```python
from build123d import *

# Parameters (mm, degrees)
BOSS_EXTRUDE1_DEPTH = 16
CUT_EXTRUDE1_DEPTH  = 16
FILLET1_R           = 0.4
FILLET2_R           = 0.4
FILLET3_R           = 0.4
FILLET4_R           = 0.4
FILLET5_R           = 6.2
FILLET6_R           = 6.2
FILLET7_R           = 6.2
FILLET8_R           = 6.2
FILLET9_R           = 0.1
FILLET10_R          = 0.1
FILLET11_R          = 0.1
FILLET12_R          = 0.1
FILLET13_R          = 0.1
FILLET14_R          = 0.1
FILLET15_R          = 0.1
FILLET16_R          = 0.1
FILLET17_R          = 0.1
FILLET18_R          = 0.1
FILLET19_R          = 0.1
FILLET20_R          = 0.1
FILLET21_R          = 0.1
FILLET22_R          = 0.1
FILLET23_R          = 0.1
FILLET24_R          = 0.1


with BuildPart() as part:
    # Sketch1 → Boss-Extrude1 (new body)
    with BuildSketch(Plane.XY):
        with BuildLine():
            Line((-1.085, -1.085), (-1.085, -2.903924069))
            ThreePointArc((-1.085, -2.903924069), (0, -3.1), (1.085, -2.903924069))
            Line((1.085, -2.903924069), (1.085, -1.085))
            Line((1.085, -1.085), (2.903924069, -1.085))
            ThreePointArc((2.903924069, -1.085), (3.1, 0), (2.903924069, 1.085))
            Line((2.903924069, 1.085), (1.085, 1.085))
            Line((1.085, 1.085), (1.085, 2.903924069))
            ThreePointArc((1.085, 2.903924069), (0, 3.1), (-1.085, 2.903924069))
            Line((-1.085, 2.903924069), (-1.085, 1.085))
            Line((-1.085, 1.085), (-2.903924069, 1.085))
            ThreePointArc((-2.903924069, 1.085), (-3.1, 0), (-2.903924069, -1.085))
            Line((-2.903924069, -1.085), (-1.085, -1.085))
        make_face()
    extrude(amount=BOSS_EXTRUDE1_DEPTH)

    # Sketch2 → Cut-Extrude1 (cut)
    with BuildSketch(Plane.XY):
        with BuildLine():
            Line((0.84, -0.84), (2.248199279, -0.84))
            ThreePointArc((2.248199279, -0.84), (2.4, 0), (2.248199279, 0.84))
            Line((2.248199279, 0.84), (0.84, 0.84))
            Line((0.84, 0.84), (0.84, 2.248199279))
            ThreePointArc((0.84, 2.248199279), (0, 2.4), (-0.84, 2.248199279))
            Line((-0.84, 2.248199279), (-0.84, 0.84))
            Line((-0.84, 0.84), (-2.248199279, 0.84))
            ThreePointArc((-2.248199279, 0.84), (-2.4, 0), (-2.248199279, -0.84))
            Line((-2.248199279, -0.84), (-0.84, -0.84))
            Line((-0.84, -0.84), (-0.84, -2.248199279))
            ThreePointArc((-0.84, -2.248199279), (0, -2.4), (0.84, -2.248199279))
            Line((0.84, -2.248199279), (0.84, -0.84))
        make_face()
    extrude(amount=CUT_EXTRUDE1_DEPTH, mode=Mode.SUBTRACT)

    # Fillet1
    fillet1_edges = [part.edges().sort_by_distance(p)[0] for p in [
        (-0.84, 0.84, 8),
    ]]
    fillet(fillet1_edges, radius=FILLET1_R)

    # Fillet2
    fillet2_edges = [part.edges().sort_by_distance(p)[0] for p in [
        (0.84, 0.84, 8),
    ]]
    fillet(fillet2_edges, radius=FILLET2_R)

    # Fillet3
    fillet3_edges = [part.edges().sort_by_distance(p)[0] for p in [
        (0.84, -0.84, 8),
    ]]
    fillet(fillet3_edges, radius=FILLET3_R)

    # Fillet4
    fillet4_edges = [part.edges().sort_by_distance(p)[0] for p in [
        (-0.84, -0.84, 8),
    ]]
    fillet(fillet4_edges, radius=FILLET4_R)

    # Fillet5
    # the kernel refuses this fillet: 6.2 mm, written as the material it adds along each edge
    with BuildSketch(Plane(origin=(-1.085, 1.085, 0), x_dir=(-1, 0, 0), z_dir=(0, 0, 1))) as fillet5_piece_1:
        with BuildLine():
            CenterArc((5.198154004, -5.198154004), FILLET5_R, 123.027198012, 23.945603977)
            Line((0, -1.818924069), (0, 0))
            Line((0, 0), (1.818924069, 0))
        make_face()
    extrude(amount=16)

    # Fillet6
    # the kernel refuses this fillet: 6.2 mm, written as the material it adds along each edge
    with BuildSketch(Plane(origin=(-1.085, -1.085, 0), x_dir=(-1, 0, 0), z_dir=(0, 0, 1))) as fillet6_piece_1:
        with BuildLine():
            CenterArc((5.198154004, 5.198154004), FILLET6_R, 213.027198012, 23.945603977)
            Line((0, 1.818924069), (0, 0))
            Line((0, 0), (1.818924069, 0))
        make_face()
    extrude(amount=16)

    # Fillet7
    # the kernel refuses this fillet: 6.2 mm, written as the material it adds along each edge
    with BuildSketch(Plane(origin=(1.085, -1.085, 0), x_dir=(0, -1, 0), z_dir=(0, 0, 1))) as fillet7_piece_1:
        with BuildLine():
            CenterArc((5.198154004, 5.198154004), FILLET7_R, 213.027198012, 23.945603977)
            Line((0, 1.818924069), (0, 0))
            Line((0, 0), (1.818924069, 0))
        make_face()
    extrude(amount=16)

    # Fillet8
    # the kernel refuses this fillet: 6.2 mm, written as the material it adds along each edge
    with BuildSketch(Plane(origin=(1.085, 1.085, 0), x_dir=(1, 0, 0), z_dir=(0, 0, 1))) as fillet8_piece_1:
        with BuildLine():
            CenterArc((5.198154004, 5.198154004), FILLET8_R, 213.027198012, 23.945603977)
            Line((0, 1.818924069), (0, 0))
            Line((0, 0), (1.818924069, 0))
        make_face()
    extrude(amount=16)

    # Fillet9
    fillet9_edges = [part.edges().sort_by_distance(p)[0] for p in [
        (0.84, 2.248199279, 8),
    ]]
    fillet(fillet9_edges, radius=FILLET9_R)

    # Fillet10
    fillet10_edges = [part.edges().sort_by_distance(p)[0] for p in [
        (1.085, 2.903924069, 8),
    ]]
    fillet(fillet10_edges, radius=FILLET10_R)

    # Fillet11
    fillet11_edges = [part.edges().sort_by_distance(p)[0] for p in [
        (-1.085, 2.903924069, 8),
    ]]
    fillet(fillet11_edges, radius=FILLET11_R)

    # Fillet12
    fillet12_edges = [part.edges().sort_by_distance(p)[0] for p in [
        (-2.903924069, 1.085, 8),
    ]]
    fillet(fillet12_edges, radius=FILLET12_R)

    # Fillet13
    fillet13_edges = [part.edges().sort_by_distance(p)[0] for p in [
        (-2.903924069, -1.085, 8),
    ]]
    fillet(fillet13_edges, radius=FILLET13_R)

    # Fillet14
    fillet14_edges = [part.edges().sort_by_distance(p)[0] for p in [
        (-1.085, -2.903924069, 8),
    ]]
    fillet(fillet14_edges, radius=FILLET14_R)

    # Fillet15
    fillet15_edges = [part.edges().sort_by_distance(p)[0] for p in [
        (1.085, -2.903924069, 8),
    ]]
    fillet(fillet15_edges, radius=FILLET15_R)

    # Fillet16
    fillet16_edges = [part.edges().sort_by_distance(p)[0] for p in [
        (2.903924069, -1.085, 8),
    ]]
    fillet(fillet16_edges, radius=FILLET16_R)

    # Fillet17
    fillet17_edges = [part.edges().sort_by_distance(p)[0] for p in [
        (2.903924069, 1.085, 8),
    ]]
    fillet(fillet17_edges, radius=FILLET17_R)

    # Fillet18
    fillet18_edges = [part.edges().sort_by_distance(p)[0] for p in [
        (0.84, -2.248199279, 8),
    ]]
    fillet(fillet18_edges, radius=FILLET18_R)

    # Fillet19
    fillet19_edges = [part.edges().sort_by_distance(p)[0] for p in [
        (-0.84, -2.248199279, 8),
    ]]
    fillet(fillet19_edges, radius=FILLET19_R)

    # Fillet20
    fillet20_edges = [part.edges().sort_by_distance(p)[0] for p in [
        (-2.248199279, 0.84, 8),
    ]]
    fillet(fillet20_edges, radius=FILLET20_R)

    # Fillet21
    fillet21_edges = [part.edges().sort_by_distance(p)[0] for p in [
        (-2.248199279, -0.84, 8),
    ]]
    fillet(fillet21_edges, radius=FILLET21_R)

    # Fillet22
    fillet22_edges = [part.edges().sort_by_distance(p)[0] for p in [
        (-0.84, 2.248199279, 8),
    ]]
    fillet(fillet22_edges, radius=FILLET22_R)

    # Fillet23
    fillet23_edges = [part.edges().sort_by_distance(p)[0] for p in [
        (2.248199279, -0.84, 8),
    ]]
    fillet(fillet23_edges, radius=FILLET23_R)

    # Fillet24
    fillet24_edges = [part.edges().sort_by_distance(p)[0] for p in [
        (2.248199279, 0.84, 8),
    ]]
    fillet(fillet24_edges, radius=FILLET24_R)


solid = part.part
```
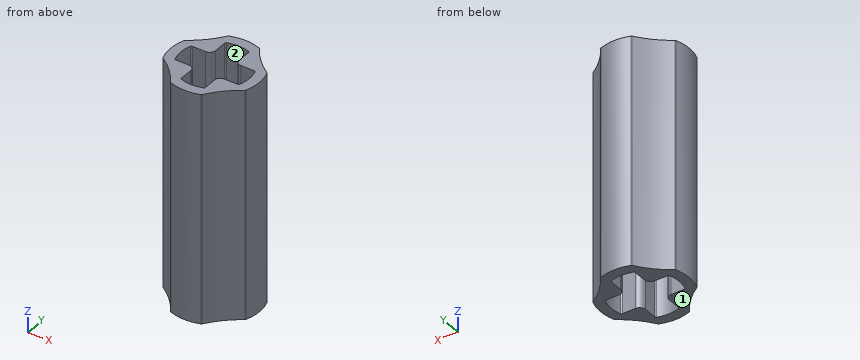
Here's how the part is built. I have some questions about the finished solid (model axes, mm). Face numbers are marked on the shaded views. A direction names the side the tool comes from. Give positions to 0.01 mm unless a question says otherwise; leave off trailing zeros. Loops run counter-clockwise (first coordinate to the right, second up) from the corner with the lowest first, then second, coordinate; pieces in that order, holes last. Notation, with made-up numbers: M 75,-29 L 130,-29 A20 ccw 130,-4 Z; hole C -27,-8.5 d4. An arc over 180 degrees is marked long. Put each result on its own line as item: value. Start each with the question number.
(1) I want a section at A-A on x = 1.75. Please give me the cut outline in (y, z), then the cut area to 3 significant figures.
(2) For the marked faces 1 and 2, which set-ups out of +Z, -Z, +X, -X, +Y, -Y let a thin tool reach every point of the face, with its end or its side?
(3) I need wall thicknesses on line 1 along X through (y, z) = (0, 5.5); line 2 along Y through (x, z) = (1.75, 7); line 3 along X through (y, z) = (1.25, 1.75). Which ranges of each line are inside material? Lowest first, please. Write a range as [from, to].
(4) Will these pins go through, and if not, where does the flat tip stop? pin 1 Ø1 at (y, z) = (1.5, 4.5) entering from -X; pin 2 Ø1 at (x, z) = (2, 8) entering from +Y; pin 3 Ø1 at (x, z) = (-2, 9) entering from -Y.
(5) I want a section at B-B on y = -0.25. Please give me the cut outline in (x, z), then the cut area to 3 significant figures.
Answer block:
1. outline: M -2.05,0 L -0.84,0 L -0.84,16 L -2.05,16 Z; M 0.84,0 L 2.05,0 L 2.05,16 L 0.84,16 Z
1. area: 38.8 mm^2
2. face 1: -Z, +X, -X, +Y, -Y
2. face 2: +Z, -Z
3. line 1: [-3.1, -2.4], [2.4, 3.1]
3. line 2: [-2.05, -0.84], [0.84, 2.05]
3. line 3: [-2.66, -0.84], [0.84, 2.66]
4. pin 1: x = -2.93
4. pin 2: y = 2.34
4. pin 3: y = -2.34
5. outline: M -3.09,0 L -2.39,0 L -2.39,16 L -3.09,16 Z; M 2.39,0 L 3.09,0 L 3.09,16 L 2.39,16 Z
5. area: 22.5 mm^2
